Autodesk Fusion 360 part; units mm, degrees
sketch "Top" plane through (0, 0, 0) normal (0, 0, 1) x (1, 0, 0)
  line L0 (0, 0) -> (40, 0)
  line L1 (40, 0) -> (40, 50)
  line L2 (40, 50) -> (0, 50)
  line L3 (0, 50) -> (0, 0)
  circle A0 centre (20, 25) radius 11.2
  circle A1 centre (20, 25) radius 6
  dimension "d6" = 40
  dimension "d7" = 50
  dimension "d11" = 22.4
  dimension "d12" = 25
  dimension "d13" = 20
  dimension "d27" = 12
extrude "Extrude1" add sketch "Top" along normal blind 10 contours L0 L1 L2 L3 | A0 | A1
extrude "Extrude2" cut sketch "Top" along normal blind 8 contours A0 | A1
extrude "Extrude5" cut sketch "Top" along normal blind 110 contours A1
sketch "Sketch3" plane through (0, 0, 0) normal (0, -1, 0) x (1, 0, 0)
  line L0 (0, 0) -> (40, 0)
  line L1 (40, 0) -> (40, 10)
  line L2 (40, 10) -> (0, 10)
  line L3 (0, 10) -> (0, 0)
  line L4 (24, 5) -> (22, 8.4641)
  line L5 (22, 8.4641) -> (18, 8.4641)
  line L6 (18, 8.4641) -> (16, 5)
  line L7 (16, 5) -> (18, 1.5359)
  line L8 (18, 1.5359) -> (22, 1.5359)
  line L9 (22, 1.5359) -> (24, 5)
  point P0 (20, 5)
  dimension "d34" = 4
  dimension "d37" = 20
  dimension "d38" = 5
extrude "Extrude6" cut sketch "Sketch3" against normal blind 5 contours L4 L5 L6 L7 L8 L9
sketch "Sketch4" plane through (0, 50, 0) normal (0, 1, 0) x (-1, 0, 0)
  line L0 (-40, 0) -> (0, 0)
  line L1 (0, 0) -> (0, 10)
  line L2 (0, 10) -> (-40, 10)
  line L3 (-40, 10) -> (-40, 0)
  line L4 (-22.8284, 7.8284) -> (-23.8637, 3.9647)
  line L5 (-23.8637, 3.9647) -> (-21.0353, 1.1363)
  line L6 (-21.0353, 1.1363) -> (-17.1716, 2.1716)
  line L7 (-17.1716, 2.1716) -> (-16.1363, 6.0353)
  line L8 (-16.1363, 6.0353) -> (-18.9647, 8.8637)
  line L9 (-18.9647, 8.8637) -> (-22.8284, 7.8284)
  point P0 (-20, 5)
  dimension "d39" = 4
  dimension "d42" = 20
  dimension "d43" = 5
extrude "Extrude7" cut sketch "Sketch4" against normal blind 5 contours L4 L5 L6 L7 L8 L9
sketch "Sketch5" plane through (0, 0, 0) normal (-1, 0, 0) x (0, -1, 0)
  line L0 (-50, 0) -> (0, 0)
  line L1 (0, 0) -> (0, 10)
  line L2 (0, 10) -> (-50, 10)
  line L3 (-50, 10) -> (-50, 0)
  line L4 (-30, 10) -> (-20, 10)
  line L5 (-20, 10) -> (-20, 0)
  line L6 (-20, 0) -> (-30, 0)
  line L7 (-30, 0) -> (-30, 10)
  dimension "d50" = 10
  dimension "d51" = 10
  dimension "d52" = 20
extrude "Extrude8" add sketch "Sketch5" along normal blind 50 contours L0 L2 L4 L5 L6 L7
sketch "Sketch7" plane through (0, 0, 10) normal (0, 0, 1) x (-1, 0, 0)
  circle A0 centre (-20, -25) radius 6
  line L0 (0, -50) -> (0, -30)
  line L1 (0, -30) -> (50, -30)
  line L2 (50, -30) -> (50, -20)
  line L3 (50, -20) -> (0, -20)
  line L4 (0, -20) -> (0, 0)
  line L5 (0, 0) -> (-40, 0)
  line L6 (-40, 0) -> (-40, -50)
  line L7 (-40, -50) -> (0, -50)
  line L8 (45, -28) -> (37, -28)
  line L9 (37, -28) -> (37, -22)
  line L10 (37, -22) -> (45, -22)
  line L11 (45, -22) -> (45, -28)
  dimension "d64" = 6
  dimension "d65" = 8
  dimension "d67" = 5
  dimension "d69" = 2
extrude "Extrude10" cut sketch "Sketch7" against normal blind 100 contours L8 L9 L10 L11
equation "length = 50 mm"
equation "width = 40 mm"
equation "thickness = 10 mm"
equation "extra = 100 mm"
equation "fit_gap = 0.2 mm"
equation "d6 = width"
equation "d7 = length"
equation "d8 = thickness"
equation "bearing_outer_radius = 11.1 mm"
equation "d11 = ( bearing_outer_radius * 2 ) + fit_gap"
equation "d12 = length / 2"
equation "d13 = width / 2"
equation "d14 = thickness - 2 mm"
equation "bearing_inner_radius = ( 8 mm + 4 mm ) / 2"
equation "d27 = bearing_inner_radius * 2"
equation "d28 = thickness + extra"
equation "polygon_dowel_hole_side_length = 4 mm"
equation "polygon_dowel_hole_side_height = 5 mm"
equation "polygon_dowel_hole_big_distance = width / 2"
equation "polygon_dowel_hole_small_distance = thickness / 2"
equation "d34 = polygon_dowel_hole_side_length"
equation "d37 = polygon_dowel_hole_big_distance"
equation "d38 = polygon_dowel_hole_small_distance"
equation "d39 = polygon_dowel_hole_side_length"
equation "d42 = polygon_dowel_hole_big_distance"
equation "d43 = polygon_dowel_hole_small_distance"
equation "ackerman_bracket_length = 50 mm"
equation "ackerman_bracket_width = 10 mm"
equation "ackerman_bracket_big_distance = ( length - ackerman_bracket_width ) / 2"
equation "d50 = ackerman_bracket_width"
equation "d51 = ackerman_bracket_width"
equation "d52 = ackerman_bracket_big_distance"
equation "d53 = ackerman_bracket_length"
equation "ackerman_bracket_dowel_length = 8 mm"
equation "ackerman_bracket_dowel_width = 6 mm"
equation "ackerman_bracket_dowel_big_distance = 5 mm"
equation "ackerman_bracket_dowel_small_distance = ( ackerman_bracket_width - ackerman_bracket_dowel_width ) / 2"
equation "d64 = ackerman_bracket_dowel_width"
equation "d65 = ackerman_bracket_dowel_length"
equation "d67 = ackerman_bracket_dowel_big_distance"
equation "d69 = ackerman_bracket_dowel_small_distance"
Could you check a few things on this model? Use its own coordinates, in mm. A direction names the side the tool comes from. Round coordinates to 2 decimals unless told otherwise and drop trailing zeros. Order: outer loops, then holes, each group sorted by start corner. A loop starts at its lowest first (then second) coordinate and runs counter-clockwise, first axis right, second up. Notation, with made-up numbers: (43.25, 22) -> (71.25, 22) arc R11 ccw to (71.25, 40) -> close; hole circle Ø1 at (-14, 47.25). An arc over 180 degrees is marked (long way). One line per question, with ' | ' between items.
Q1. If I drill on line 1 (X direction, y = 25, z = 9.1); line 2 (Y direction, x = 20, z = 5.5); line 3 (Y direction, x = -43.5, z = 6), over which ranges is the centre line in solid material (lowest first)? Write a range as from..to.
Computed values:
line 1: -50..-45, -37..14, 26..40 | line 2: 5..13.8, 36.2..45 | line 3: 20..22, 28..30
Q2. Which directions (+Z, -Z, +X, -X, +Y, -Y) give clear straight access to the entire face, cutting with the end or side of a thin tool? Please do faces 1 (the face through (-41, 22, 5)), 2 (the face through (25, 20, 8)), 3 (the face through (0, 40, 5)), 4 (the face through (20, 2, 8.464)), 5 (the face through (23.34, 47.54, 5.92)).
Computed values:
face 1: +Z, -Z | face 2: -Z | face 3: +Z, -Z, -X, +Y | face 4: -Y | face 5: +Y
Q3. I'm going to push flat-ended pins straight in: pin 1 (3 mm diameter, centred on x = -16, z = 7, fed in from +Y); pin 2 (3 mm diameter, centred on y = 5.5, z = 6.5, fed in from -X); pin 3 (18 mm diameter, centred on x = 25.5, y = 30, fed in from -Z); pin 4 (5 mm diameter, centred on x = -28, z = 6, fed in from -Y). Where does each tip first touch, or does it pass through?
Computed values:
pin 1: y = 30 | pin 2: x = 0 | pin 3: z = 0 | pin 4: y = 20
Q4. We'd pull the mould along Z, two halves only. Please class faces 6 (the face through (20.87, 47.535, 8.353)), 7 (the face through (-50, 25, 5)), 8 (the face through (4, 25, 0)): released by +Z, released by -Z, zero draft, split by the parting line, or undercut.
Computed values:
face 6: undercut | face 7: zero draft | face 8: released by -Z
Q5. If we section it at C-C on y = 16.5: Write out the boundary of the cut face in (x, z).
Computed values:
outline: (0, 0) -> (12.71, 0) -> (12.71, 8) -> (27.29, 8) -> (27.29, 0) -> (40, 0) -> (40, 10) -> (0, 10) -> close
Q6. If we section it at A-A on y = 25: Write out the boundary of the cut face in (x, z), plus the area to 3 significant figures.
Computed values:
outline: (-50, 0) -> (-45, 0) -> (-45, 10) -> (-50, 10) -> close; (-37, 0) -> (8.8, 0) -> (8.8, 8) -> (14, 8) -> (14, 10) -> (-37, 10) -> close; (26, 8) -> (31.2, 8) -> (31.2, 0) -> (40, 0) -> (40, 10) -> (26, 10) -> close | area: 617 mm²
Q7. If we section it at B-B on x = 20: Write out the boundary of the cut face in (y, z), plus the area to 3 significant figures.
Computed values:
outline: (0, 0) -> (13.8, 0) -> (13.8, 8) -> (19, 8) -> (19, 10) -> (0, 10) -> (0, 8.46) -> (5, 8.46) -> (5, 1.54) -> (0, 1.54) -> close; (31, 8) -> (36.2, 8) -> (36.2, 0) -> (50, 0) -> (50, 1.41) -> (45, 1.41) -> (45, 8.59) -> (50, 8.59) -> (50, 10) -> (31, 10) -> close | area: 226 mm²
Q8. If we section it at D-D on x = -16: Write out the boundary of the cut face in (y, z), plus the area to 3 significant figures.
Computed values:
outline: (20, 0) -> (30, 0) -> (30, 10) -> (20, 10) -> close | area: 100 mm²
